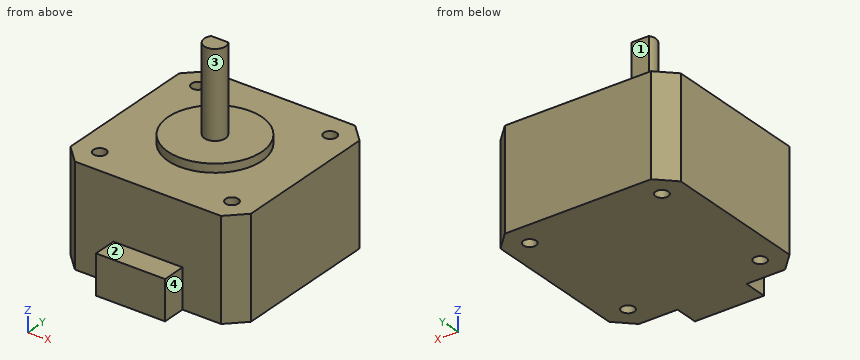
```python
from build123d import *

# Parameters (mm, degrees)
SKETCH1_R           = 1.5
BOSS_EXTRUDE1_DEPTH = 23.5
SKETCH2_W           = 16.2
SKETCH2_H           = 9.2
BOSS_EXTRUDE2_DEPTH = 5.5
SKETCH3_R           = 11
BOSS_EXTRUDE3_DEPTH = 2
SKETCH4_R           = 2.5
BOSS_EXTRUDE4_DEPTH = 20
SKETCH5_W           = 5
SKETCH5_H           = 18
CUT_EXTRUDE1_DEPTH  = 1


with BuildPart() as part:
    # Sketch1 → Boss-Extrude1 (new body)
    with BuildSketch(Plane.XY):
        Polygon((-17.15, -21.15), (17.15, -21.15), (21.15, -17.15), (21.15, 17.15), (17.15, 21.15), (-17.15, 21.15), (-21.15, 17.15), (-21.15, -17.15), align=None)
        with Locations((-15.5, 15.5)):
            Circle(SKETCH1_R, mode=Mode.SUBTRACT)
        with Locations((15.5, 15.5)):
            Circle(SKETCH1_R, mode=Mode.SUBTRACT)
        with Locations((15.5, -15.5)):
            Circle(SKETCH1_R, mode=Mode.SUBTRACT)
        with Locations((-15.5, -15.5)):
            Circle(SKETCH1_R, mode=Mode.SUBTRACT)
    extrude(amount=BOSS_EXTRUDE1_DEPTH)

    # Sketch2 → Boss-Extrude2 (add)
    with BuildSketch(Plane.XZ.offset(21.15)):
        with Locations((0, 4.6)):
            Rectangle(SKETCH2_W, SKETCH2_H)
    extrude(amount=BOSS_EXTRUDE2_DEPTH)

    # Sketch3 → Boss-Extrude3 (add)
    with BuildSketch(Plane.XY.offset(23.5)):
        with Locations(Location((0, 0, 0), (0, 0, 180))):
            Circle(SKETCH3_R)
    extrude(amount=BOSS_EXTRUDE3_DEPTH)

    # Sketch4 → Boss-Extrude4 (add)
    with BuildSketch(Plane.XY.offset(25.5)):
        Circle(SKETCH4_R)
    extrude(amount=BOSS_EXTRUDE4_DEPTH)

    # Sketch5 → Cut-Extrude1 (cut)
    with BuildSketch(Plane(origin=(0, 2.5, 0), x_dir=(1, 0, 0), z_dir=(0, 1, 0))):
        with Locations((0, -36.5)):
            Rectangle(SKETCH5_W, SKETCH5_H)
    extrude(amount=-CUT_EXTRUDE1_DEPTH, mode=Mode.SUBTRACT)


solid = part.part
```
Can you work these out from the model? Positions are in its coordinate system, mm. Face numbers are marked on the shaded views. A direction names the side the tool comes from. Coordinates: 2 decimals unless noted, no trailing zeros. Loops run counter-clockwise (first coordinate to the right, second up) from the corner with the lowest first, then second, coordinate; pieces in that order, holes last. Notation, with made-up numbers: (71, -26.5) - (82, -26.5) arc R17 cw to (82, -10.5) - close; hole circle Ø4 at (60.25, -24). An arc over 180 degrees is marked (long way). Use a Markdown table: item, result.
Item 1: For the marked faces 1, 2, 3 and 4, which set-ups out of +Z, -Z, +X, -X, +Y, -Y let a thin tool reach every point of the face, with its end or its side?
Numbers:
| item | result |
|---|---|
| face 1 | +Z, +X, -X, +Y |
| face 2 | +Z, +X, -X, -Y |
| face 3 | +Z |
| face 4 | +Z, -Z, +X, -Y |
Item 2: If I drill on probe 1 along Y at (x, z) = (15.5, 17.5); probe 2 along X at (y, z) = (-15, 17), over which ranges is the centre line in solid material (lowest first)? Write a range as from..to.
Numbers:
| item | result |
|---|---|
| probe 1 | y = -21.15..-17, -14..14, 17..21.15 |
| probe 2 | x = -21.15..-16.91, -14.09..14.09, 16.91..21.15 |
Item 3: Will these pins go through, and if not, where does the flat tip stop? pin 1 (2 mm diameter, centred on x = 1, z = 34, fed in from +Y); pin 2 (2 mm diameter, centred on x = 12.5, y = -21.5, fed in from +Z); pin 3 (1.6 mm diameter, centred on y = -25, z = 5.5, fed in from +X).
Numbers:
| item | result |
|---|---|
| pin 1 | stops at y = 1.5 |
| pin 2 | stops at z = 23.5 |
| pin 3 | stops at x = 8.1 |
Item 4: I want a section at A-A on y = -15.5. Please give me the cut outline in (x, z), and give its area (3 significant figures).
Numbers:
| item | result |
|---|---|
| outline | (-21.15, 0) - (-17, 0) - (-17, 23.5) - (-21.15, 23.5) - close; (-14, 0) - (14, 0) - (14, 23.5) - (-14, 23.5) - close; (17, 0) - (21.15, 0) - (21.15, 23.5) - (17, 23.5) - close |
| area | 853 mm2 |
Item 5: I want a section at C-C on z = 21. Please give me the cut outline in (x, y), and give its area (3 significant figures).
Numbers:
| item | result |
|---|---|
| outline | (-21.15, -17.15) - (-17.15, -21.15) - (17.15, -21.15) - (21.15, -17.15) - (21.15, 17.15) - (17.15, 21.15) - (-17.15, 21.15) - (-21.15, 17.15) - close; hole circle Ø3 at (-15.5, -15.5); hole circle Ø3 at (-15.5, 15.5); hole circle Ø3 at (15.5, -15.5); hole circle Ø3 at (15.5, 15.5) |
| area | 1,730 mm2 |
Item 6: I want a section at D-D on y = 0. Please give me the cut outline in (x, z).
Numbers:
| item | result |
|---|---|
| outline | (-21.15, 0) - (21.15, 0) - (21.15, 23.5) - (11, 23.5) - (11, 25.5) - (2.5, 25.5) - (2.5, 45.5) - (-2.5, 45.5) - (-2.5, 25.5) - (-11, 25.5) - (-11, 23.5) - (-21.15, 23.5) - close |
